Autodesk Inventor part; units mm, degrees
ref_plane "YZ Plane" through (0, 0, 0) normal (1, 0, 0) x (0, 1, 0)
ref_plane "XZ Plane" through (0, 0, 0) normal (0, 1, 0) x (-1, 0, 0)
ref_plane "XY Plane" through (0, 0, 0) normal (0, 0, 1) x (1, 0, 0)
sketch "スケッチ1" plane through (0, 0, 0) normal (0, 1, 0) x (-1, 0, 0)
  circle A0 centre (0, 0) radius 10
  dimension "d0" = 20
extrude "押し出し2" add sketch "スケッチ1" along normal blind 1.5
sketch "スケッチ3" plane through (0, 0, 0) normal (0, -1, 0) x (1, 0, 0)
  circle A0 centre (0, 0) radius 10
  circle A1 centre (0, 0) radius 2
  dimension "d21" = 4
hole "穴2" at (0, 0, 0) direction (0, 1, 0) diameter 4 end through all counterbore diameter 10 counterbore depth 1
sketch "スケッチ4" plane through (0, 0, 0) normal (0, -1, 0) x (1, 0, 0)
  circle A0 centre (0, 0) radius 5
  circle A1 centre (0, 7) radius 1
  dimension "d30" = 0
  dimension "d31" = 7
  dimension "d32" = 2
hole "穴3" at (0, 0, 7) direction (0, 1, 0) diameter 2.1 end through all
pattern_circular "円形状パターン2" count 8 over 360 about axis through (0, 0.5, 0) along (0, -1, 0) of "穴3"
properties part number "13" material "アセタール樹脂、白"
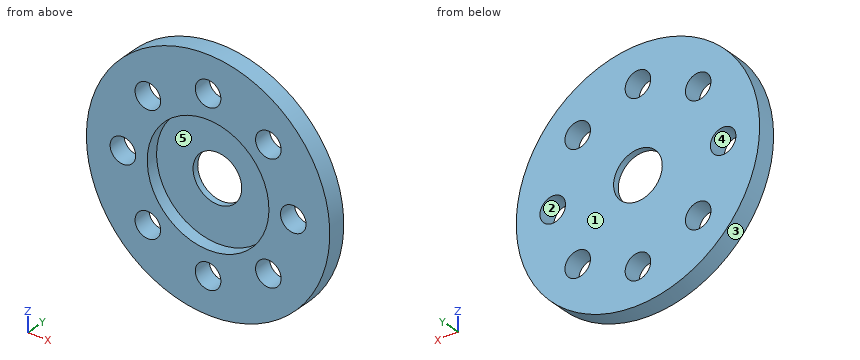
Can you work these out from the model? Positions are in its coordinate system, mm. Face numbers are marked on the shaded views. A direction names the side the tool comes from. Give positions to 0.01 mm unless a question says otherwise; leave off trailing zeros. Loops run counter-clockwise (first coordinate to the right, second up) from the corner with the lowest first, then second, coordinate; pieces in that order, holes last. Notation, with made-up numbers: (61, -26.5) -> (79, -26.5) arc R10 cw to (79, -7.5) -> close; hole circle Ø7 at (67.5, 21.5). An arc over 180 degrees is marked (long way). Return JSON: item names as keys, results as strings.
Q1. We'd pull the mould along X, two halves only. Please class the marked faces 1, 2 and 3: released by +X, released by -X, zero draft, split by the parting line, or undercut.
Checks:
{"face 1": "zero draft", "face 2": "undercut", "face 3": "split by the parting line"}
Q2. On a 3-axis mill with a long thin cutter (end or side, diameter ignored), from which of +Z, -Z, +X, -X, +Y, -Y can I reach the whole of each face in a straight line? I mean the marked faces 4 and 5. Say none if no direction works.
Checks:
{"face 4": "+Y, -Y", "face 5": "-Y"}
Q3. I want a section at D-D, the plane z = -6.5. List the corners of the cut face in (x, y) for me.
Checks:
{"outline": "(-7.6, 0) -> (-0.92, 0) -> (-0.92, 1.5) -> (-7.6, 1.5) -> close; (0.92, 0) -> (7.6, 0) -> (7.6, 1.5) -> (0.92, 1.5) -> close"}
Q4. I want a section at A-A, the plane x = 0. List the corners of the cut face in (y, z) for me, then the cut area to 3 significant figures.
Checks:
{"outline": "(0, -10) -> (1.5, -10) -> (1.5, -8.05) -> (0, -8.05) -> close; (0, -5.95) -> (1.5, -5.95) -> (1.5, -2) -> (1, -2) -> (1, -5) -> (0, -5) -> close; (0, 5) -> (1, 5) -> (1, 2) -> (1.5, 2) -> (1.5, 5.95) -> (0, 5.95) -> close; (0, 8.05) -> (1.5, 8.05) -> (1.5, 10) -> (0, 10) -> close", "area": "11.7 mm2"}
Q5. I want a section at B-B, the plane z = 0. List the corners of the cut face in (x, y) for me, then the cut area to 3 significant figures.
Checks:
{"outline": "(-10, 0) -> (-8.05, 0) -> (-8.05, 1.5) -> (-10, 1.5) -> close; (-5.95, 0) -> (-5, 0) -> (-5, 1) -> (-2, 1) -> (-2, 1.5) -> (-5.95, 1.5) -> close; (2, 1) -> (5, 1) -> (5, 0) -> (5.95, 0) -> (5.95, 1.5) -> (2, 1.5) -> close; (8.05, 0) -> (10, 0) -> (10, 1.5) -> (8.05, 1.5) -> close", "area": "11.7 mm2"}
Q6. I want a section at C-C, the plane x = -6.75. List the corners of the cut face in (y, z) for me, then the cut area to 3 significant figures.
Checks:
{"outline": "(0, -7.38) -> (1.5, -7.38) -> (1.5, -1.02) -> (0, -1.02) -> close; (0, 1.02) -> (1.5, 1.02) -> (1.5, 7.38) -> (0, 7.38) -> close", "area": "19.1 mm2"}
Q7. For pin 1 Ø1.9 at (x, z) = (0, -7) entering from +Y; pin 2 Ø9 at (x, z) = (0, 0) entering from +Y; pin 3 Ø3 at (x, z) = (1.5, 0) entering from -Y, each with a flat end and sliding along its axis, tell me the tip position at first contact or that it passes through.
Checks:
{"pin 1": "passes through", "pin 2": "stops at y = 1.5", "pin 3": "stops at y = 1"}
Q8. I need wall thicknesses on probe 1 along X at (y, z) = (0.3, 5.25); probe 2 along Z at (x, y) = (-5.5, 1.4); probe 3 along X at (y, z) = (0.3, -6.25). Which ranges of each line are inside material? Lowest first, please.
Checks:
{"probe 1": "x = -8.51 to -5.96, -3.94 to 3.94, 5.96 to 8.51", "probe 2": "z = -8.35 to -5.84, -4.06 to 4.06, 5.84 to 8.35", "probe 3": "x = -7.81 to -0.73, 0.73 to 7.81"}
